Source: CAD feature listing. Evaluate the final solid. Frame: model axes, mm. Face numbers are marked on the shaded views. A direction names the side the tool comes from. Round coordinates to 2 decimals unless told otherwise and drop trailing zeros. Write each loop counter-clockwise with the first axis right and the second up, starting at its lowest first coordinate (ties: lowest second). Pieces come first, ordered by that corner, then holes. Notation, with made-up numbers: M -1,58 L 24,58 A26 cw 24,80 Z; hole C 2,-35.5 d3. An arc over 180 degrees is marked long. Answer in a Markdown table with one row per item.
Solid Edge part; units mm, degrees
sketch "Sketch1" plane through (0, 0, 0) normal (0, -1, 0) x (1, 0, 0)
  line L0 (-84.6631, 66.5335) -> (-44.6631, 66.5335)
  line L1 (-44.6631, 66.5335) -> (-44.6631, -63.4665)
  line L2 (-44.6631, -63.4665) -> (-84.6631, -63.4665)
  line L3 (-84.6631, -63.4665) -> (-84.6631, -58.4665)
  line L4 (-84.6631, -58.4665) -> (-49.6631, -58.4665)
  line L5 (-49.6631, -58.4665) -> (-49.6631, 61.5335)
  line L6 (-49.6631, 61.5335) -> (-84.6631, 61.5335)
  line L7 (-84.6631, 61.5335) -> (-84.6631, 66.5335)
  dimension "D1" = 44.6631
  dimension "D2" = 84.6631
  dimension "D3" = 84.6631
  dimension "D4" = 44.6631
extrude "Protrusion1" add sketch "Sketch1" along normal blind 240
sketch "Sketch2" plane through (-49.6631, -60, 1.5335) normal (-1, 0, 0) x (0, -1, 0)
  circle A0 centre (120, 0) radius 7.5
  dimension "D1" = 120
extrude "Cutout1" cut sketch "Sketch2" against normal through all
properties material "Aluminum, 6061-T6"
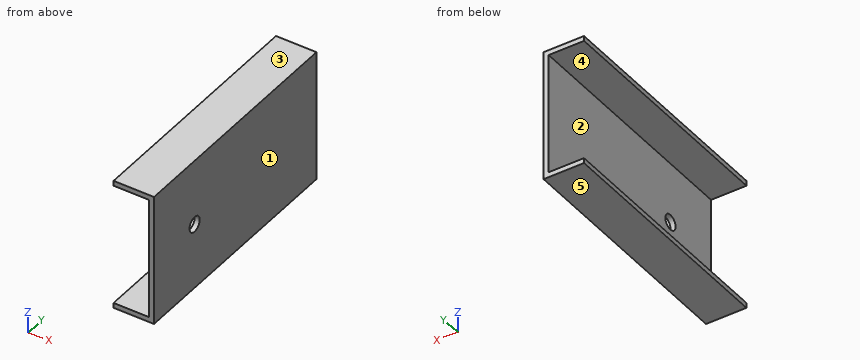
Q1. Contact query for flat-ended pins moving along their axis: pin 1 Ø1.5 at (y, z) = (-198.5, 3) entering from -X; pin 2 Ø2 at (y, z) = (-184, 4) entering from -X. Output: stop coordinate, or through.
Solutions:
| item | result |
|---|---|
| pin 1 | stops at x = -49.66 |
| pin 2 | passes through |
Q2. Section B-B (x = -63). Return loops of the section in (y, z).
Solutions:
| item | result |
|---|---|
| outline | M -240,-63.47 L 0,-63.47 L 0,-58.47 L -240,-58.47 Z; M -240,61.53 L 0,61.53 L 0,66.53 L -240,66.53 Z |
Q3. Section A-A (y = -180). Return loops of the section in (x, z).
Solutions:
| item | result |
|---|---|
| outline | M -84.66,-63.47 L -44.66,-63.47 L -44.66,-5.97 L -49.66,-5.97 L -49.66,-58.47 L -84.66,-58.47 Z; M -84.66,61.53 L -49.66,61.53 L -49.66,9.03 L -44.66,9.03 L -44.66,66.53 L -84.66,66.53 Z |
Q4. Material intervals for probe 1 along Z at (x, y) = (-54.5, -24); probe 2 along Z at (x, y) = (-48, -180); probe 3 along X at (y, z) = (-70, 18), sorted ascending.
Solutions:
| item | result |
|---|---|
| probe 1 | z = -63.47 to -58.47, 61.53 to 66.53 |
| probe 2 | z = -63.47 to -5.97, 9.03 to 66.53 |
| probe 3 | x = -49.66 to -44.66 |
Q5. Access query for the marked faces 4 and 5. Directions: +Z, -Z, +X, -X, +Y, -Y. A direction counts if a zero-diameter tool reaches every point of the face in a straight line with its end or side. Return the directions, or none.
Solutions:
| item | result |
|---|---|
| face 4 | -X, +Y, -Y |
| face 5 | -Z, +X, -X, +Y, -Y |
Q6. Section C-C (y = -61). Return loops of the section in (x, z).
Solutions:
| item | result |
|---|---|
| outline | M -84.66,-63.47 L -44.66,-63.47 L -44.66,66.53 L -84.66,66.53 L -84.66,61.53 L -49.66,61.53 L -49.66,-58.47 L -84.66,-58.47 Z |
Q7. Section D-D (z = 33.5). Return loops of the section in (x, y), and give its area (3 significant figures).
Solutions:
| item | result |
|---|---|
| outline | M -49.66,-240 L -44.66,-240 L -44.66,0 L -49.66,0 Z |
| area | 1,200 mm2 |
Q8. Pull-direction query (Z, two-part tool) for the marked faces 1, 2 and 3; classes: pulls with the +Z half, pulls with the -Z half, needs draft (parallel to the pull), parting line crosses it, or undercut.
Solutions:
| item | result |
|---|---|
| face 1 | needs draft |
| face 2 | undercut |
| face 3 | pulls with the +Z half |
